The model under review builds one solid part; all positions refer to its coordinate system, in mm. Round coordinates to 2 decimals unless told otherwise and drop trailing zeros. Order: outer loops, then holes, each group sorted by start corner. A loop starts at its lowest first (then second) coordinate and runs counter-clockwise, first axis right, second up.
1) Consider section C-C (x = 45). Give the boundary of the cut face in (y, z).
2) Consider section A-A (z = 25). Give the boundary of the cut face in (x, y), then the cut area to 3 significant figures.
3) To check wall thickness, follow L1, parallel to Z at x = 25, y = -4.5; L2, parallel to Z at x = 7, y = -6.75; L3, parallel to Z at x = 36.5, y = -2.25. State the ranges of each line that lie inside material, in increasing order.
4) Consider section B-B (y = -6.5). Give the boundary of the cut face in (x, z).
5) Clearance check with flat-ended pins moving along their axes: P1, Ø1, axis at y = -4, z = 411, coming from the -X side; P2, Ø1, axis at x = 41.5, y = -4, coming from the +Z side; P3, Ø13, axis at x = 25, z = 25, coming from the +Y side. State where each tip first meets the part, or that it passes through.
from build123d import *

# Parameters (mm, degrees)
F1_DEPTH = 8
F3_D     = 16
F4_R     = 10
F6_DEPTH = 25


with BuildPart() as f1:
    # F0 (on Front) → F1 (new body)
    with BuildSketch(Plane.XZ):
        with BuildLine():
            Line((0, 105.297409), (0, 0))
            Line((0, 0), (50, 0))
            Line((50, 0), (50, 600))
            Line((50, 600), (0, 600))
            Line((0, 600), (0, 243.861474))
            ThreePointArc((0, 243.861474), (20, 174.579442), (0, 105.297409))
        make_face()
    extrude(amount=F1_DEPTH)

    # F3 (through all)
    with Locations(Plane.XZ.offset(8)):
        with Locations((25, 25)):
            Hole(F3_D / 2)

    # F4
    f4_edges = [f1.edges().sort_by_distance(p)[0] for p in [
        (0, -4, 0),
    ]]
    fillet(f4_edges, radius=F4_R)

    # F5 (on face) → F6 (cut)
    with BuildSketch(Plane.XZ.offset(8)):
        Polygon((50, 600), (25, 600), (50, 539.896909), align=None)
    extrude(amount=-F6_DEPTH, mode=Mode.SUBTRACT)


solid = f1.part
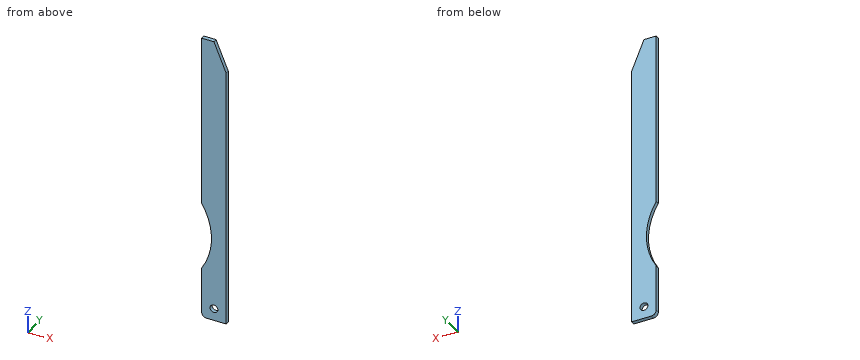
Answer below:
1. outline: (-8, 0) - (0, 0) - (0, 551.92) - (-8, 551.92) - close
2. outline: (0, -8) - (17, -8) - (17, 0) - (0, 0) - close; (33, -8) - (50, -8) - (50, 0) - (33, 0) - close
2. area: 272 mm2
3. L1: z = 0 to 17, 33 to 600
3. L2: z = 0.46 to 117.91, 231.25 to 600
3. L3: z = 0 to 572.35
4. outline: (0, 10) arc R10 ccw to (10, 0) - (50, 0) - (50, 539.9) - (25, 600) - (0, 600) - (0, 243.86) arc R130 cw to (0, 105.3) - close; hole circle Ø16 at (25, 25)
5. P1: stops at x = 0
5. P2: stops at z = 561.53
5. P3: passes through
